```python
from build123d import *

# Parameters (mm, degrees)
CYLINDER_R        = 0.4
CYLINDER_DEPTH    = 1
FILLET_R          = 0.8
CYLINDER002_R     = 0.4
CYLINDER002_DEPTH = 0.6
CYLINDER001_R     = 0.65
CYLINDER001_DEPTH = 0.6
CHAMFER_SIZE      = 0.2


with BuildPart() as cylinder:
    # Cylinder → Cylinder (new body)
    with BuildSketch(Plane.XY):
        Circle(CYLINDER_R)
    extrude(amount=CYLINDER_DEPTH)


with BuildPart() as cone001:
    # Cone001 → Cone001 (revolve)
    with BuildSketch(Plane.XZ):
        Polygon((0, 0), (14, 0), (13.8, 1), (0, 1), align=None)
    revolve(axis=Axis((0, 0, 0), (0, 0, 1)))


with BuildPart() as fillet_body:
    # Cone → Cone (revolve)
    with BuildSketch(Plane.XZ):
        Polygon((0, 0), (13.8, 0), (14, 1), (0, 1), align=None)
    revolve(axis=Axis((0, 0, 0), (0, 0, 1)))

    # Fusion: union Cone001
    add(cone001.part)

    # Cut: cut Cylinder
    add(cylinder.part, mode=Mode.SUBTRACT)

    # Fillet
    fillet_edges = [fillet_body.edges().sort_by_distance(p)[0] for p in [
        (-0.4, 0, 0),
    ]]
    fillet(fillet_edges, radius=FILLET_R)


with BuildPart() as cylinder002:
    # Cylinder002 → Cylinder002 (new body)
    with BuildSketch(Plane.XY.offset(1)):
        Circle(CYLINDER002_R)
    extrude(amount=CYLINDER002_DEPTH)


with BuildPart() as fusion001:
    # Cylinder001 → Cylinder001 (new body)
    with BuildSketch(Plane.XY.offset(1)):
        Circle(CYLINDER001_R)
    extrude(amount=CYLINDER001_DEPTH)

    # Cut001: cut Cylinder002
    add(cylinder002.part, mode=Mode.SUBTRACT)

    # Chamfer
    chamfer_edges = [fusion001.edges().sort_by_distance(p)[0] for p in [
        (-0.65, 0, 1.6),
    ]]
    chamfer(chamfer_edges, length=CHAMFER_SIZE)

    # Fusion001: union Fillet body
    add(fillet_body.part)


solid = fusion001.part
```
Source: CAD feature listing. Evaluate the final solid. Frame: model axes, mm. A direction names the side the tool comes from. Round coordinates to 2 decimals unless told otherwise and drop trailing zeros. Loops run counter-clockwise (first coordinate to the right, second up) from the corner with the lowest first, then second, coordinate; pieces in that order, holes last. Notation, with made-up numbers: M 73,72 L 79,72 A16 ccw 79,83 Z; hole C 73.5,-26 d9. An arc over 180 degrees is marked long. Put each result on its own line as item: value.
(1) Section A-A, the plane y = 0. Return loops of the section in (x, z).
Solutions:
outline: M -14,0 L -1.2,0 A0.8 ccw -0.4,0.8 L -0.4,1.6 L -0.45,1.6 L -0.65,1.4 L -0.65,1 L -14,1 L -13.9,0.5 Z; M 0.4,0.8 A0.8 ccw 1.2,0 L 14,0 L 13.9,0.5 L 14,1 L 0.65,1 L 0.65,1.4 L 0.45,1.6 L 0.4,1.6 Z
(2) First-contact query: pin 1 (10 mm diameter, centred on x = 4, y = 4, fed in from -Z); pin 2 (8.5 mm diameter, centred on x = 6, y = -4.5, fed in from +Z). Flat tips, straight axial feed; report the tip coordinate or a pass-through.
Solutions:
pin 1: z = 0
pin 2: z = 1
(3) Ray query, line 1 (Y direction, x = 0, z = 1.1); line 2 (Z direction, x = 2.5, y = 7.5); line 3 (Y direction, x = 0, z = 0.55). Return the intervals inside material, ascending. Write a range as [from, to].
Solutions:
line 1: [-0.65, -0.4], [0.4, 0.65]
line 2: [0, 1]
line 3: [-13.91, -0.44], [0.44, 13.91]
(4) Access query for faces 1 (the face through (0, -3, 0)), 2 (the face through (-0.085, 0.644, 1.197)). Directions: +Z, -Z, +X, -X, +Y, -Y. A direction counts if a zero-diameter tool reaches every point of the face in a straight line with its end or side. Return the directions, or none.
Solutions:
face 1: -Z, +X, -X, +Y, -Y
face 2: +Z
